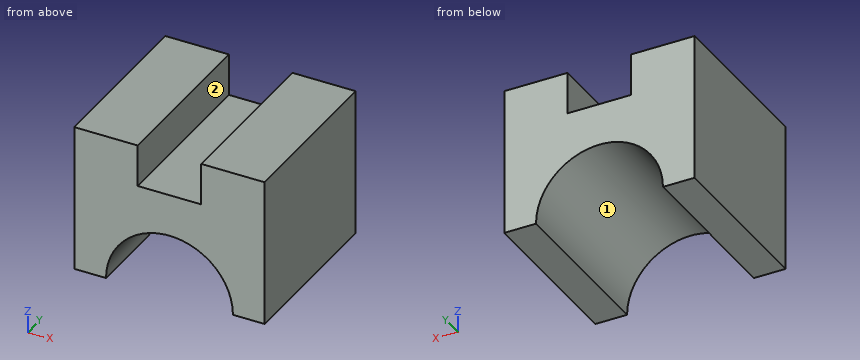
```python
from build123d import *

# Parameters (mm, degrees)
F0_W     = 114.3
F0_H     = 101.6
F1_DEPTH = 63.5
F2_W     = 38.1
F2_H     = 101.6
F3_DEPTH = 25.4
F5_D     = 76.2


with BuildPart() as f1:
    # F0 (on Top) → F1 (new body)
    with BuildSketch(Plane.XY):
        with Locations((57.15, 50.8)):
            Rectangle(F0_W, F0_H)
    extrude(amount=F1_DEPTH)

    # F2 (on face) → F3 (join)
    with BuildSketch(Plane.XY.offset(63.5)):
        with Locations((19.05, 50.8)):
            Rectangle(F2_W, F2_H)
        with Locations((95.25, 50.8)):
            Rectangle(F2_W, F2_H)
    extrude(amount=F3_DEPTH)

    # F5 (through all)
    with Locations(Plane.XZ):
        with Locations((57.15, 0)):
            Hole(F5_D / 2)


solid = f1.part
```
Read the model definition and answer for the solid it produces. Units are mm, in the model's axes. Face numbers are marked on the shaded views. A direction names the side the tool comes from. Give positions to 0.01 mm unless a question says otherwise; leave off trailing zeros. Order: outer loops, then holes, each group sorted by start corner. A loop starts at its lowest first (then second) coordinate and runs counter-clockwise, first axis right, second up. Notation, with made-up numbers: (8.25, -11) -> (24.25, -11) arc R23 cw to (24.25, 9) -> close; hole circle Ø3 at (54.5, 60.25). An arc over 180 degrees is marked (long way). Write item = value, one per line.
1. A cutting plane is placed at C-C, the plane x = 57.15. Write down the section's boundary in (y, z).
Numbers:
outline = (0, 38.1) -> (101.6, 38.1) -> (101.6, 63.5) -> (0, 63.5) -> close
2. Straight lines are drawn through the part: line 1 along X through (y, z) = (86, 82); line 2 along X through (y, z) = (62.5, 7.5); line 3 along Z through (x, y) = (74.5, 68). For each, find the intervals that lie inside material, in ascending order.
Numbers:
line_1 = 0 to 38.1, 76.2 to 114.3
line_2 = 0 to 19.8, 94.5 to 114.3
line_3 = 33.92 to 63.5
3. A cutting plane is placed at D-D, the plane z = 20. Write down the section's boundary in (x, y).
Numbers:
outline = (0, 0) -> (24.72, 0) -> (24.72, 101.6) -> (0, 101.6) -> close; (89.58, 0) -> (114.3, 0) -> (114.3, 101.6) -> (89.58, 101.6) -> close
4. Given pin 1 (1.5 mm diameter, centred on x = 38, y = 88, fed in from -Z), flat-ended and moving along its own axis, determine where the tip first touches the part or whether it passes through.
Numbers:
pin_1 = 32.49
5. For the marked faces 1 and 2, determine the directions among +Z, -Z, +X, -X, +Y, -Y from which every point of the face is accessible in a straight line to the end or side of a thin tool.
Numbers:
face_1 = -Z, +Y, -Y
face_2 = +Z, +Y, -Y
6. A cutting plane is placed at A-A, the plane z = 69. Write down the section's boundary in (x, y), and give its area (3 significant figures).
Numbers:
outline = (0, 0) -> (38.1, 0) -> (38.1, 101.6) -> (0, 101.6) -> close; (76.2, 0) -> (114.3, 0) -> (114.3, 101.6) -> (76.2, 101.6) -> close
area = 7,740 mm²
7. A cutting plane is placed at B-B, the plane y = 61. Write down the section's boundary in (x, z).
Numbers:
outline = (0, 0) -> (19.05, 0) arc R38.1 cw to (95.25, 0) -> (114.3, 0) -> (114.3, 88.9) -> (76.2, 88.9) -> (76.2, 63.5) -> (38.1, 63.5) -> (38.1, 88.9) -> (0, 88.9) -> close
